Design review of the part shown in the three views and the two pictorial views. Dimensions are in mm from the part's minimum x, y and z. A direction names the side the tool comes from. Coordinates: 2 decimals unless noted, no trailing zeros. Write each loop counter-clockwise with the first axis right and the second up, starting at its lowest first coordinate (ties: lowest second). Pieces come first, ordered by that corner, then holes. Notation, with made-up numbers: (62, 15) -> (88, 15) arc R29 ccw to (88, 53) -> close; hole circle Ø1 at (-38, 52). An arc over 180 degrees is marked (long way). Answer in a Markdown table with one row per item. Add a question column.
Item 1: Clearance check with flat-ended pins moving along their axes: P1, Ø8, axis at x = 30, z = 5.5, coming from the -Y side; P2, Ø3, axis at x = 67.5, y = 32, coming from the +Z side; P3, Ø7.5, axis at x = 11.5, z = 41.5, coming from the +Y side. State where each tip first meets the part, or that it passes through.
Item 2: Draft analysis for pull direction X (two halves, no side actions). For the marked faces 1, 2 and 3, state which applies: released by +X, released by -X, zero draft, split by the parting line, or undercut.
Item 3: Take a section at B-B, the plane z = 14.5. Write out the cut boundary in (x, y).
Item 4: Take a section at C-C, the plane x = 8.5. Write out the cut boundary in (y, z).
Item 5: Take a section at D-D, the plane y = 39.5. Write out the cut boundary in (x, z), and give its area (3 significant figures).
Item 6: Take a section at A-A, the plane y = 22. Write out the cut boundary in (x, z), and give its area (3 significant figures).
Item 7: To check wall thickness, follow line 1 (X direction, y = 9.5, z = 14); line 2 (Z direction, x = 64.5, y = 40.5). State the ranges of each line that lie inside material, in increasing order.
Item 8: For the marked faces 4, 5, 6, 7 and 8, list the 3-axis set-ups (+Z, -Z, +X, -X, +Y, -Y) from which the entire face can be reached by the end or side of a thin tool; tool diameter is ignored.
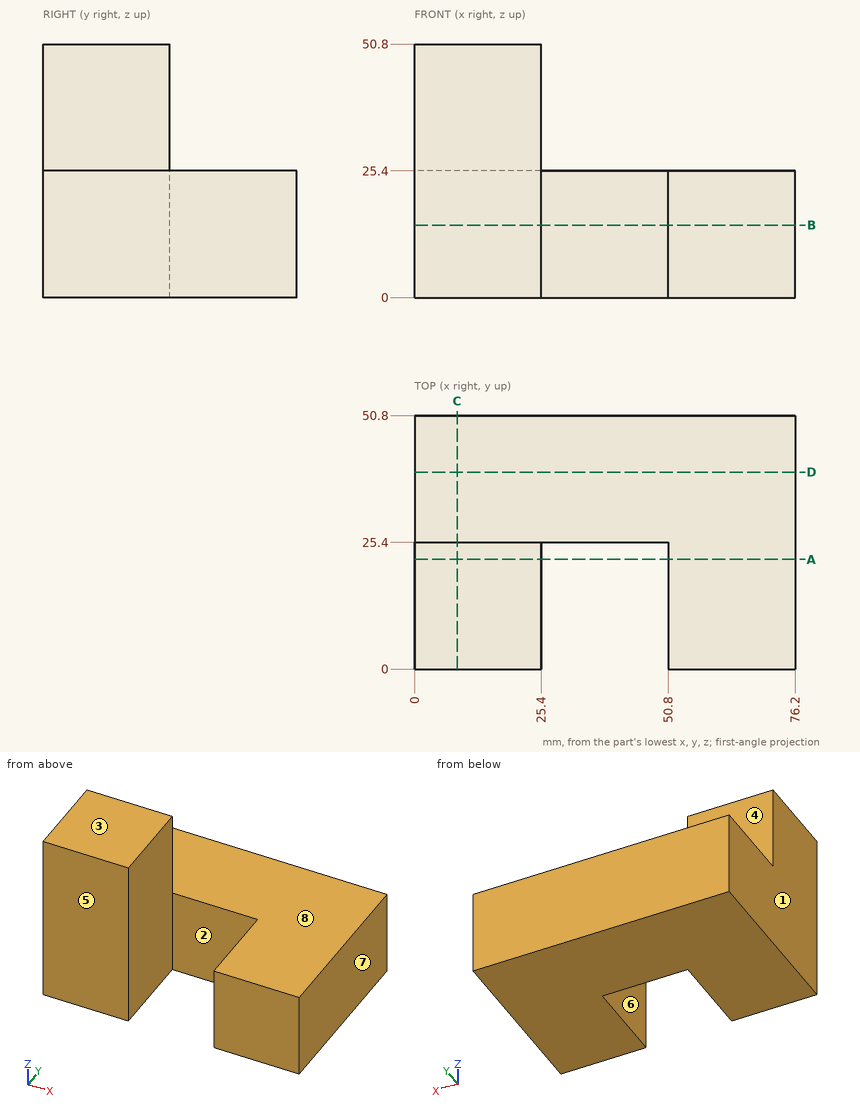
Answers:
| question | item | result |
|---|---|---|
| 1 | P1 | stops at y = 25.4 |
| 1 | P2 | stops at z = 25.4 |
| 1 | P3 | stops at y = 25.4 |
| 2 | face 1 | released by -X |
| 2 | face 2 | undercut |
| 2 | face 3 | zero draft |
| 3 | outline | (0, 0) -> (25.4, 0) -> (25.4, 25.4) -> (50.8, 25.4) -> (50.8, 0) -> (76.2, 0) -> (76.2, 50.8) -> (0, 50.8) -> close |
| 4 | outline | (0, 0) -> (50.8, 0) -> (50.8, 25.4) -> (25.4, 25.4) -> (25.4, 50.8) -> (0, 50.8) -> close |
| 5 | outline | (0, 0) -> (76.2, 0) -> (76.2, 25.4) -> (0, 25.4) -> close |
| 5 | area | 1,940 mm^2 |
| 6 | outline | (0, 0) -> (25.4, 0) -> (25.4, 50.8) -> (0, 50.8) -> close; (50.8, 0) -> (76.2, 0) -> (76.2, 25.4) -> (50.8, 25.4) -> close |
| 6 | area | 1,940 mm^2 |
| 7 | line 1 | x = 0 to 25.4, 50.8 to 76.2 |
| 7 | line 2 | z = 0 to 25.4 |
| 8 | face 4 | +Z, +X, -X, +Y |
| 8 | face 5 | +Z, -Z, +X, -X, -Y |
| 8 | face 6 | +Z, -Z, -Y |
| 8 | face 7 | +Z, -Z, +X, +Y, -Y |
| 8 | face 8 | +Z, +X, +Y |
